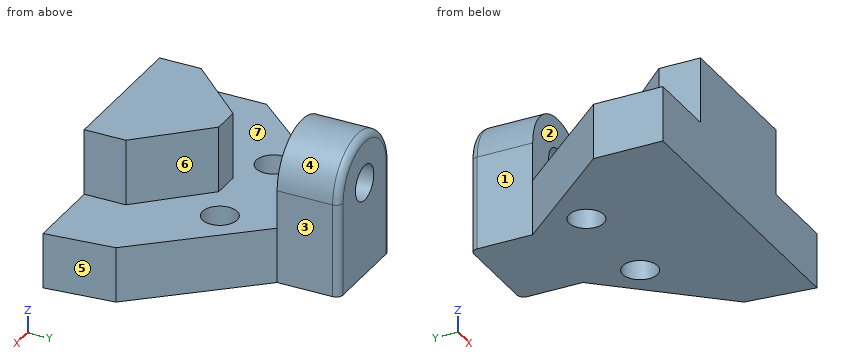
```python
from build123d import *

# Parameters (mm, degrees)
EXTRUDE_1_DEPTH         = 16
EXTRUDE_2_DEPTH         = 19
EXTRUDE_3_DEPTH         = 18
FILLET_1_R              = 2
HOLE_WIZARD_M12_1_D     = 10.2
HOLE_WIZARD_M12_1_DEPTH = 18
HOLE_WIZARD_10_0_10_1_D = 10


with BuildPart() as part:
    # 草图1 → 凸台-拉伸1 (new body)
    with BuildSketch(Plane.XY):
        Polygon((14, 32), (-14, 32), (-42, 0), (-42, -20), (44, -20), (42, 0), align=None)
    extrude(amount=EXTRUDE_1_DEPTH)

    # 草图2 → 凸台-拉伸2 (add)
    with BuildSketch(Plane.XY.offset(16)):
        Polygon((4, 10), (-4, 10), (-21, -8), (-21, -20), (21, -20), (21, -8), align=None)
    extrude(amount=EXTRUDE_2_DEPTH)

    # 草图5 → 凸台-拉伸3 (add)
    with BuildSketch(Plane(origin=(0, 32, 0), x_dir=(1, 0, 0), z_dir=(0, 1, 0))):
        with BuildLine():
            Line((-14, 0), (-14, -27))
            ThreePointArc((-14, -27), (0, -41), (14, -27))
            Line((14, -27), (14, 0))
            Line((14, 0), (-14, 0))
        make_face()
    extrude(amount=EXTRUDE_3_DEPTH)

    # 圆角1
    fillet_1_edges = [part.edges().sort_by_distance(p)[0] for p in [
        (0, 50, 41),
        (14, 50, 13.5),
        (-14, 50, 13.5),
    ]]
    fillet(fillet_1_edges, radius=FILLET_1_R)

    # M12 螺纹孔1
    with Locations(Plane(origin=(0, 50, 0), x_dir=(1, 0, 0), z_dir=(0, 1, 0))):
        with Locations((0, -27)):
            Hole(HOLE_WIZARD_M12_1_D / 2, depth=HOLE_WIZARD_M12_1_DEPTH)

    # Ø10.0 (10) 直径孔1 (through all)
    with Locations(Plane.XY.offset(16)):
        with Locations((-15, 16), (15, 16)):
            Hole(HOLE_WIZARD_10_0_10_1_D / 2)


solid = part.part
```
Geometry check sheet. Reference: the model listing, model coordinates, mm. Face numbers are marked on the shaded views. A direction names the side the tool comes from. Round coordinates to 2 decimals unless told otherwise and drop trailing zeros. Loops run counter-clockwise (first coordinate to the right, second up) from the corner with the lowest first, then second, coordinate; pieces in that order, holes last. Notation, with made-up numbers: (13.5, 21) - (47.5, 21) arc R27 cw to (47.5, 45) - close; hole circle Ø11 at (52.25, 2). An arc over 180 degrees is marked (long way). Write each question's results on one line, items separated by ' | '. Start each with the question number.
Q1. Cross-section at C-C on y = 16. Enter the section's corners in (x, z).
Q2. Cross-section at D-D on y = -9. Enter the section's corners in (x, z), and give its area (3 significant figures).
Q3. Access from +Z, -Z, +X, -X, +Y, -Y to the whole of each face (thin tool, end or side, straight path). Record for the marked faces 1, 2 and 3.
Q4. Cross-section at B-B on x = 0. Enter the section's corners in (y, z), and give its area (3 significant figures).
Q5. Thickness scan on line 1 (Z direction, x = 0, y = 43); line 2 (X direction, y = 45, z = 27); line 3 (X direction, y = 17.5, z = 15). Record the ranges inside material, lowest first. Write a range as [from, to].
Q6. Cross-section at A-A on z = 3. Enter the section's corners in (x, y), and give its area (3 significant figures).
Q7. Release check for a two-part mould opening along Y. For the marked faces 4, 5, 6 and 7 record: +Y half, -Y half, draft (parallel to the pull), parting line (faces both ways), or undercut.
Q8. Gauge pin test, flat ends, axial feed: P1, Ø1, axis at y = 9.5, z = 27.5, coming from the +X side; P2, Ø6, axis at y = -11, z = 25.5, coming from the +X side; P3, Ø6, axis at y = -3, z = 23.5, coming from the -X side. Record the tip position at first contact, or that the pin passes through.
Answers below:
1) outline: (-28, 0) - (-20, 0) - (-20, 16) - (-28, 16) - close; (-10, 0) - (10, 0) - (10, 16) - (-10, 16) - close; (20, 0) - (28, 0) - (28, 16) - (20, 16) - close
2) outline: (-42, 0) - (42.9, 0) - (42.9, 16) - (21, 16) - (21, 35) - (-21, 35) - (-21, 16) - (-42, 16) - close | area: 2,160 mm²
3) face 1: +Z, -Z, -X, +Y | face 2: +Z, +X, -X | face 3: +Z, -Z, +X, +Y
4) outline: (-20, 0) - (50, 0) - (50, 21.9) - (32, 21.9) - (32, 16) - (10, 16) - (10, 35) - (-20, 35) - close; (32, 32.1) - (50, 32.1) - (50, 39) arc R2 ccw to (48, 41) - (32, 41) - close | area: 1,960 mm²
5) line 1: z = [0, 21.9], [32.1, 41] | line 2: x = [-14, -5.1], [5.1, 14] | line 3: x = [-26.69, -19.77], [-10.23, 10.23], [19.77, 26.69]
6) outline: (-42, -20) - (44, -20) - (42, 0) - (14, 32) - (14, 48) arc R2 ccw to (12, 50) - (-12, 50) arc R2 ccw to (-14, 48) - (-14, 32) - (-42, 0) - close; hole circle Ø10 at (-15, 16); hole circle Ø10 at (15, 16) | area: 3,840 mm²
7) face 4: draft | face 5: +Y half | face 6: undercut | face 7: undercut
8) P1: stops at x = 4.94 | P2: stops at x = 21 | P3: stops at x = -19.11
